Check sheet for the drawn part. Datum: minimum x, y, z corner. Units: mm. A direction names the side the tool comes from. Give positions to 0.01 mm unless a question says otherwise; leave off trailing zeros. Write each loop counter-clockwise with the first axis right and the second up, starting at its lowest first coordinate (ties: lowest second). Pieces come first, ordered by that corner, then holes. Notation, with made-up numbers: (-14, -38) - (10, -38) arc R25 cw to (10, 0) - close; hole circle Ø1 at (-27.75, 42). An arc over 180 degrees is marked (long way). Answer as a JSON object with one key per item and string values. Group by question number.
Item 1: Go/stop test with flat-tipped pins: pin 1 (2 mm diameter, centred on x = 1.5, y = 6, fed in from +Z); pin 2 (4 mm diameter, centred on y = 6, z = 10.5, fed in from +X); pin 3 (3 mm diameter, centred on y = 3.5, z = 3, fed in from -X). Record where each tip stops, or that it passes through.
Item 2: Sectioned sample at A-A, the plane z = 8. Record the boundary of the cut face in (x, y).
Item 3: Tool access check on the marked faces 1, 2 and 3. Record the directions out of +Z, -Z, +X, -X, +Y, -Y that give a thin tool (end or side, any length) a straight path to the whole face; none if there is none.
Item 4: Sectioned sample at B-B, the plane y = 5. Record the boundary of the cut face in (x, z).
Item 5: Scan lines: line 1 along Y through (x, z) = (2.5, 6); line 2 along X through (y, z) = (8.5, 9.5); line 3 along X through (y, z) = (8.5, 8.25). Record each from-to range of solid material in increasing order. Write a range as [from, to].
Item 6: Sectioned sample at C-C, the plane y = 14. Record the boundary of the cut face in (x, z).
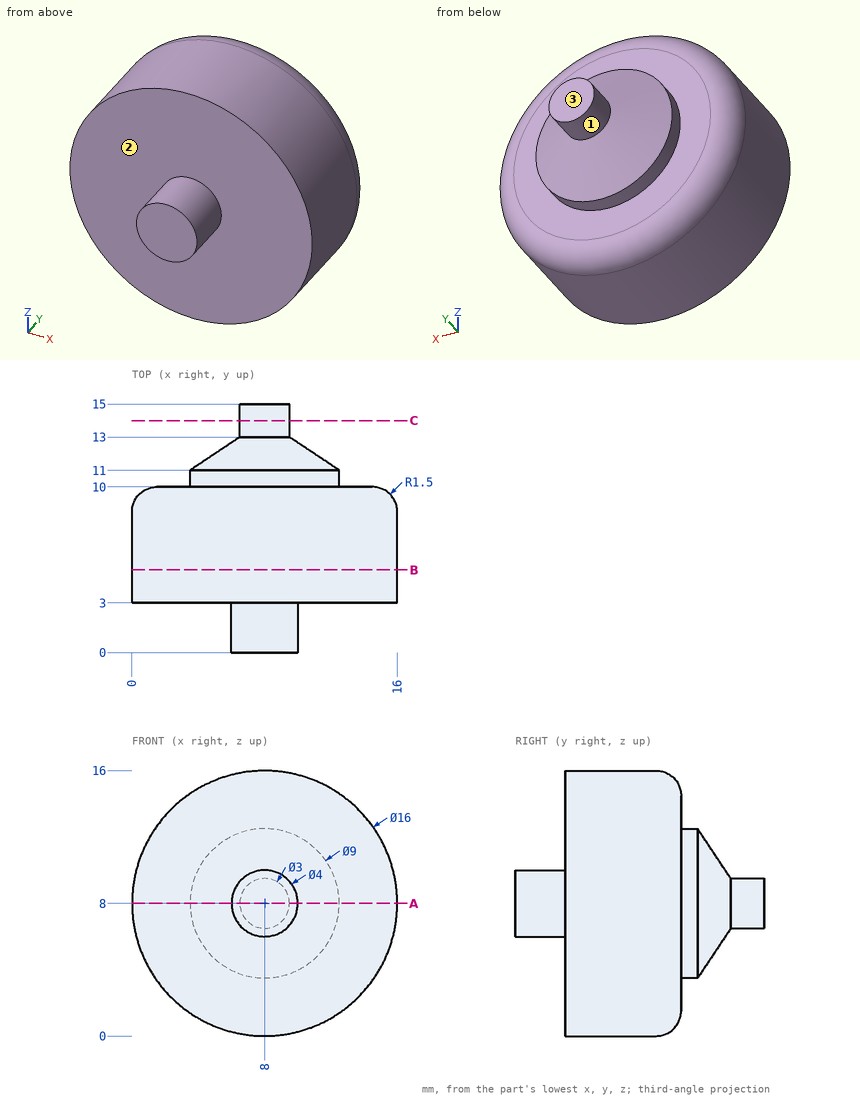
Geometry check:
{
 "1": {"pin 1": "z = 13.81", "pin 2": "x = 15.98", "pin 3": "x = 0.81"},
 "2": {"outline": "(0, 3) - (6, 3) - (6, 0) - (10, 0) - (10, 3) - (16, 3) - (16, 8.5) arc R1.5 ccw to (14.5, 10) - (12.5, 10) - (12.5, 11) - (9.5, 13) - (9.5, 15) - (6.5, 15) - (6.5, 13) - (3.5, 11) - (3.5, 10) - (1.5, 10) arc R1.5 ccw to (0, 8.5) - close"},
 "3": {"face 1": "+Y", "face 2": "-Y", "face 3": "+Z, -Z, +X, -X, +Y"},
 "4": {"outline": "circle Ø16 at (8, 8)"},
 "5": {"line 1": "[3, 10]", "line 2": "[0.14, 15.86]", "line 3": "[0, 16]"},
 "6": {"outline": "circle Ø3 at (8, 8)"}
}
